Work out the finished part from the listing and answer in its coordinate system (mm). A direction names the side the tool comes from. Give positions to 0.01 mm unless a question says otherwise; leave off trailing zeros. Write each loop counter-clockwise with the first axis right and the second up, starting at its lowest first coordinate (ties: lowest second). Pieces come first, ordered by that corner, then holes.
1) Given pin 1 Ø1.2 at (x, y) = (2.5, 0) entering from +Z; pin 2 Ø1 at (x, z) = (2, 10.5) entering from +Y, each flat-ended and moving along its own axis, determine where each tip first touches the part or whether it passes through.
2) Find section D-D (y = -1). Determine the outline of the cut face in (x, z).
3) Find section A-A (x = -1.25). Determine the outline of the cut face in (y, z), plus the area to 3 significant figures.
4) Straight lines are drawn through the part: probe 1 along X at (y, z) = (0.75, 13); probe 2 along X at (y, z) = (0, 5.5); probe 3 along Y at (x, z) = (-2.5, 1.25). For each, find the intervals that lie inside material, in ascending order.
5) A tool of negligible diameter and unlimited length cuts with its end or side. For faces 1 (the face through (3.3, 0.5, 17.5)), 2 (the face through (3, -1, 20)), from which of +Z, -Z, +X, -X, +Y, -Y can it reach the whole face along a straight path? Write none if from no direction.
6) Find section B-B (y = 0.25). Count the separate pieces of the cut face and the enclosed holes in it, plus the area to 3 significant figures.
7) Determine the mould class of faces 3 (the face through (0, -4, 9)), 4 (the face through (2.57, 1.75, 17.02)), 5 (the face through (5, 0, 9)) for opening direction X: pulls with the +X half, pulls with the -X half, needs draft (parallel to the pull), parting line crosses it, or undercut.
```python
from build123d import *

# Parameters (mm, degrees)
SKETCH_W        = 10
SKETCH_H        = 8
PAD_DEPTH       = 18
SKETCH001_R     = 1.75
PAD001_DEPTH    = 2
SKETCH002_R     = 0.75
POCKET_DEPTH    = 21
POCKET001_DEPTH = 10
POCKET002_DEPTH = 5


with BuildPart() as part:
    # Sketch → Pad (new body)
    with BuildSketch(Plane.XY):
        Rectangle(SKETCH_W, SKETCH_H)
    extrude(amount=PAD_DEPTH)

    # Sketch001 (on Face6 of Pad) → Pad001 (join)
    with BuildSketch(Plane.XY.offset(18)):
        with Locations((-2.55, 0)):
            Circle(SKETCH001_R)
        with Locations((2.55, 0)):
            Circle(SKETCH001_R)
    extrude(amount=PAD001_DEPTH)

    # Sketch002 (on Face4 of Pad001) → Pocket (cut)
    with BuildSketch(Plane(origin=(0, 0, -0.1), x_dir=(1, 0, 0), z_dir=(0, -0.052336, -0.99863))):
        with Locations((-2.55, 0)):
            Circle(SKETCH002_R)
        with Locations((2.55, 0)):
            Circle(SKETCH002_R)
    extrude(amount=-POCKET_DEPTH, mode=Mode.SUBTRACT)

    # Sketch003 (on Face2 of Pocket) → Pocket001 (cut)
    with BuildSketch(Plane(origin=(-5, 0, 0), x_dir=(0, -1, 0), z_dir=(-1, 0, 0))):
        Polygon((-4, 18), (-4, 9), (-1.7, 18), align=None)
    extrude(amount=-POCKET001_DEPTH, mode=Mode.SUBTRACT)

    # Sketch007 (on Face14 of Pocket001) → Pocket002 (cut)
    with BuildSketch(Plane.XY.offset(20)):
        with BuildLine():
            ThreePointArc((-3.3, 0), (-2.55, -0.75), (-1.8, 0))
            Line((-1.8, 0), (-1.8, 1))
            ThreePointArc((-1.8, 1), (-2.55, 1.75), (-3.3, 1))
            Line((-3.3, 0), (-3.3, 1))
        make_face()
        with BuildLine():
            ThreePointArc((1.8, 0), (2.55, -0.75), (3.3, 0))
            Line((3.3, 0), (3.3, 1))
            ThreePointArc((3.3, 1), (2.55, 1.75), (1.8, 1))
            Line((1.8, 0), (1.8, 1))
        make_face()
    extrude(amount=-POCKET002_DEPTH, mode=Mode.SUBTRACT)


solid = part.part
```
Results:
1. pin 1: stops at z = 15
1. pin 2: stops at y = 3.74
2. outline: (-5, 0) - (5, 0) - (5, 18) - (3.99, 18) - (3.99, 20) - (1.11, 20) - (1.11, 18) - (-1.11, 18) - (-1.11, 20) - (-3.99, 20) - (-3.99, 18) - (-5, 18) - close
3. outline: (-4, 0) - (4, 0) - (4, 9) - (1.7, 18) - (1.17, 18) - (1.17, 20) - (-1.17, 20) - (-1.17, 18) - (-4, 18) - close
3. area: 138 mm2
4. probe 1: x = -5 to -3.3, -1.8 to 1.8, 3.3 to 5
4. probe 2: x = -5 to -3.24, -1.86 to 1.86, 3.24 to 5
4. probe 3: y = -4 to -0.68, 0.82 to 4
5. face 1: +Z
5. face 2: +Z, +X, -X, +Y, -Y
6. separate pieces: 3
6. enclosed holes: 0
6. area: 137 mm2
7. face 3: needs draft
7. face 4: undercut
7. face 5: pulls with the +X half
